```python
from build123d import *

# Parameters (mm, degrees)
F0_W     = 26
F0_H     = 6
F1_DEPTH = 20
F2_W     = 23
F2_H     = 4
F3_DEPTH = 18
F4_R     = 2


with BuildPart() as f1:
    # F0 (on Top) → F1 (new body)
    with BuildSketch(Plane.XY):
        Rectangle(F0_W, F0_H)
    extrude(amount=F1_DEPTH)

    # F2 (on face) → F3 (cut)
    with BuildSketch(Plane.XY.offset(20)):
        Rectangle(F2_W, F2_H)
    extrude(amount=-F3_DEPTH, mode=Mode.SUBTRACT)

    # F4
    f4_edges = [f1.edges().sort_by_distance(p)[0] for p in [
        (-13, 3, 10),
        (-13, -3, 10),
        (0, -3, 0),
        (13, 0, 0),
        (0, 3, 0),
        (-13, 0, 0),
        (13, -3, 10),
        (13, 3, 10),
    ]]
    fillet(f4_edges, radius=F4_R)


solid = f1.part
```
The model under review builds one solid part; all positions refer to its coordinate system, in mm. A direction names the side the tool comes from. Coordinates: 2 decimals unless noted, no trailing zeros. Order: outer loops, then holes, each group sorted by start corner. A loop starts at its lowest first (then second) coordinate and runs counter-clockwise, first axis right, second up. Notation, with made-up numbers: (55, 60) -> (112, 60) arc R20 ccw to (112, 74) -> close; hole circle Ø9 at (-6.75, 75.5). An arc over 180 degrees is marked (long way). Answer in a Markdown table with one row per item. Add a question column.
Item 1: We need section C-C on y = 0.25. Write out the cut boundary in (x, z), plus the area to 3 significant figures.
Item 2: Clearance check with a flat-ended pin moving along its axis: pin 1 (2 mm diameter, centred on x = 3, y = -0.5, fed in from +Z). State where the tip first meets the part, or that it passes through.
Item 3: We need section A-A on z = 2.5. Write out the cut boundary in (x, y).
Item 4: We need section B-B on x = -2.25. Write out the cut boundary in (y, z), plus the area to 3 significant figures.
Item 5: Mouldability with a two-part tool opening along Y and no side actions: class faces 3 (the flat face through (0, 0, 2)), 4 (the cylindrical face through (-12.43, 2.4, 11.13)), 5 (the flat face through (0, -2, 11)), 6 (the flat face through (13, 0, 11)) as +Y half, -Y half, draft (parallel to the pull), parting line (faces both ways), or undercut.
Item 6: To check wall thickness, follow probe 1 along Y at (x, z) = (9.5, 4.5); probe 2 along X at (y, z) = (-0.75, 14.25); probe 3 along Z at (x, y) = (-10.75, -1). State the ranges of each line that lie inside material, in increasing order.
Item 7: Machinability: for faces 1 (the cylindrical face through (-12.43, 0.01, 0.6)), 2 (the flat face through (-11.5, 0, 11)), which of the approach directions +Z, -Z, +X, -X, +Y, -Y give a long, thin tool a straight path to every point of the face, cutting with its end or side? Answer none if there is none.
Final values:
| question | item | result |
|---|---|---|
| 1 | outline | (-13, 2) arc R2 ccw to (-11, 0) -> (11, 0) arc R2 ccw to (13, 2) -> (13, 20) -> (11.5, 20) -> (11.5, 2) -> (-11.5, 2) -> (-11.5, 20) -> (-13, 20) -> close |
| 1 | area | 104 mm2 |
| 2 | pin 1 | stops at z = 2 |
| 3 | outline | (-13, -1) arc R2 ccw to (-11, -3) -> (11, -3) arc R2 ccw to (13, -1) -> (13, 1) arc R2 ccw to (11, 3) -> (-11, 3) arc R2 ccw to (-13, 1) -> close; hole (-11.5, -2) -> (11.5, -2) -> (11.5, 2) -> (-11.5, 2) -> close |
| 4 | outline | (-3, 2) arc R2 ccw to (-1, 0) -> (1, 0) arc R2 ccw to (3, 2) -> (3, 20) -> (2, 20) -> (2, 2) -> (-2, 2) -> (-2, 20) -> (-3, 20) -> close |
| 4 | area | 46.3 mm2 |
| 5 | face 3 | undercut |
| 5 | face 4 | +Y half |
| 5 | face 5 | undercut |
| 5 | face 6 | draft |
| 6 | probe 1 | y = -3 to -2, 2 to 3 |
| 6 | probe 2 | x = -13 to -11.5, 11.5 to 13 |
| 6 | probe 3 | z = 0 to 2 |
| 7 | face 1 | -Z, -X, +Y, -Y |
| 7 | face 2 | +Z |
